Could you check a few things on this model? Use its own coordinates, in mm. A direction names the side the tool comes from. Round coordinates to 2 decimals unless told otherwise and drop trailing zeros. Loops run counter-clockwise (first coordinate to the right, second up) from the corner with the lowest first, then second, coordinate; pieces in that order, holes last. Notation, with made-up numbers: (13, 88) - (20, 88) arc R22 ccw to (20, 95) - close; hole circle Ø6 at (-5.75, -9). An arc over 180 degrees is marked (long way). Answer as CSV lines item,"result". Start each with the question number.
1) Suppose I cut it at C-C, the plane y = 9. Write out the boundary of the cut face in (x, z) (1 decimal), then the cut area to 3 significant figures.
2) I'm going to push flat-ended pins straight in: pin 1 Ø1 at (x, y) = (-18.5, 7.5) entering from -Z; pin 2 Ø13 at (x, z) = (0, 0) entering from +Y; pin 3 Ø2 at (y, z) = (11, -15.5) entering from -X. Where does each tip first touch, or does it pass through?
3) Which directions (+Z, -Z, +X, -X, +Y, -Y) give clear straight access to the entire face, cutting with the end or side of a thin tool? Please do faces 1 (the face through (0, 0, -5)), 2 (the face through (-7, 12.468, 7)), 3 (the face through (-30.995, 0.626, 6.883)).
4) Suppose I cut it at D-D, the plane y = 3.75. Write out the boundary of the cut face in (x, z) (1 decimal), then the cut area to 3 significant figures.
5) Please list where these lines run through material, in increasing order: line 1 along X through (y, z) = (14.6, 0); line 2 along X through (y, z) = (8.25, 0); line 3 along Z through (x, y) = (-7, 13).
6) We'd pull the mould along X, two halves only. Please class faces 4 (the face through (-13.237, 10.733, -42.034)), 5 (the face through (-1, 15.24, -19)), 6 (the face through (-10.05, 13.87, -13.1)): pulls with the +X half, pulls with the -X half, needs draft (parallel to the pull), parting line crosses it, or undercut.
```python
from build123d import *

# Parameters (mm, degrees)
SKETCH1_R           = 44.069
BOSS_EXTRUDE1_DEPTH = 15.24
SKETCH3_R           = 16.51
CUT_EXTRUDE1_DEPTH  = 2.771775
SKETCH4_R           = 4.1275
CUT_EXTRUDE2_DEPTH  = 64.557927567
BOSS_EXTRUDE2_START = 1.778
SKETCH5_R           = 9.398
SKETCH5_R_2         = 4.1275
BOSS_EXTRUDE2_DEPTH = 1.778
FILLET1_R           = 6.35
SKETCH6_R           = 31.75
SKETCH6_R_2         = 24.765
CUT_EXTRUDE3_DEPTH  = 1.27


with BuildPart() as part:
    # Sketch1 → Boss-Extrude1 (new body)
    with BuildSketch(Plane(origin=(0, 0, 0), x_dir=(1, 0, 0), z_dir=(0, 1, 0))):
        with Locations(Location((0, 0, 0), (0, 0, 90))):
            Circle(SKETCH1_R)
    extrude(amount=BOSS_EXTRUDE1_DEPTH)

    # Sketch3 → Cut-Extrude1 (cut)
    with BuildSketch(Plane(origin=(0, 15.24, 0), x_dir=(1, 0, 0), z_dir=(0, 1, 0))):
        with Locations(Location((0, 0, 0), (0, 0, 270))):
            Circle(SKETCH3_R)
    extrude(amount=-CUT_EXTRUDE1_DEPTH, mode=Mode.SUBTRACT)

    # Sketch4 → Cut-Extrude2 (cut, through all)
    with BuildSketch(Plane(origin=(0, 12.468225, 0), x_dir=(1, 0, 0), z_dir=(0, 1, 0))):
        with Locations(Location((0, 0, 0), (0, 0, 270))):
            Circle(SKETCH4_R)
    extrude(amount=-CUT_EXTRUDE2_DEPTH, mode=Mode.SUBTRACT)

    # Sketch5 → Boss-Extrude2 (add)
    with BuildSketch(Plane(origin=(0, 12.468225, 0), x_dir=(1, 0, 0), z_dir=(0, 1, 0)).offset(BOSS_EXTRUDE2_START)):
        with Locations(Location((0, 0, 0), (0, 0, 270))):
            Circle(SKETCH5_R)
        with Locations(Location((0, 0, 0), (0, 0, 270))):
            Circle(SKETCH5_R_2, mode=Mode.SUBTRACT)
    extrude(amount=-BOSS_EXTRUDE2_DEPTH)

    # Fillet1
    fillet1_edges = [part.edges().sort_by_distance(p)[0] for p in [
        (0, 0, 44.069),
    ]]
    fillet(fillet1_edges, radius=FILLET1_R)

    # Sketch6 → Cut-Extrude3 (cut)
    with BuildSketch(Plane.XZ):
        with Locations(Location((0, 0, 0), (0, 0, 270))):
            Circle(SKETCH6_R)
        with Locations(Location((0, 0, 0), (0, 0, 270))):
            Circle(SKETCH6_R_2, mode=Mode.SUBTRACT)
    extrude(amount=-CUT_EXTRUDE3_DEPTH, mode=Mode.SUBTRACT)


solid = part.part
```
Filled sheet:
1,outline,"circle Ø88.1 at (0, 0); hole circle Ø8.3 at (0, 0)"
1,area,"6,050 mm²"
2,pin 1,"z = -40.23"
2,pin 2,"y = 14.25"
2,pin 3,"x = -41.62"
3,face 1,"+Z, -Z, +X, -X, -Y"
3,face 2,"+Y"
3,face 3,"-Y"
4,outline,"circle Ø87 at (0, 0); hole circle Ø8.3 at (0, 0)"
4,area,"5,890 mm²"
5,line 1,"-44.07 to -16.51, 16.51 to 44.07"
5,line 2,"-44.07 to -4.13, 4.13 to 44.07"
5,line 3,"-43.51 to -14.95, -6.27 to 6.27, 14.95 to 43.51"
6,face 4,"parting line crosses it"
6,face 5,"needs draft"
6,face 6,"undercut"
